Part model, mm, in its own coordinate system. Face numbers are marked on the shaded views. Give positions to 0.01 mm unless a question says otherwise; leave off trailing zeros. Order: outer loops, then holes, each group sorted by start corner. A loop starts at its lowest first (then second) coordinate and runs counter-clockwise, first axis right, second up. Notation, with made-up numbers: (88.25, 4) -> (102.25, 4) arc R23 cw to (102.25, 28) -> close; hole circle Ø9 at (79, 31.5). An arc over 180 degrees is marked (long way). Write item = value, one per line. Start each with the question number.
Item 1: Band-saw the part on D-D on z = 0. Write the cut outline in (x, y).
Item 2: Band-saw the part on A-A on x = -22. Write the cut outline in (y, z), plus the area to 4 significant figures.
Item 3: Pull direction Z, two halves, no side cores. Call the marked faces 1, 2, 3 and 4: +Z half, -Z half, draft (parallel to the pull), parting line (faces both ways), or undercut.
Item 4: Band-saw the part on C-C on y = -1.75. Write the cut outline in (x, z), plus the area to 3 significant figures.
Item 5: Band-saw the part on B-B on z = 37.5. Write the cut outline in (x, y).
Item 6: Drill centre lines: line 1 along X through (y, z) = (2.4, 0); line 2 along X through (y, z) = (0.75, 37.5); line 3 along Z through (x, y) = (-30, -4.5). Where is each one in solid material? Low to high.
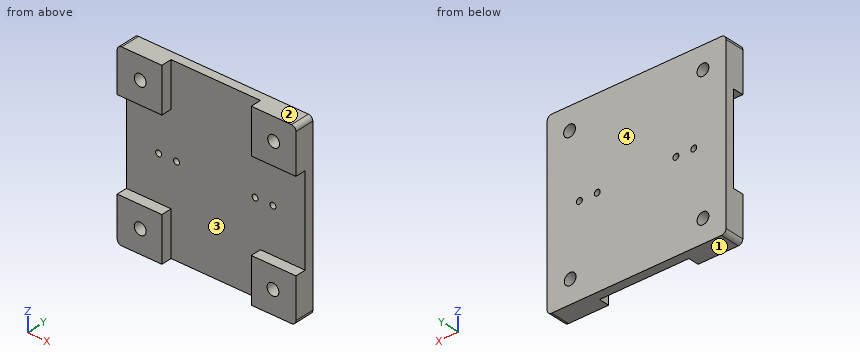
```python
from build123d import *

# Parameters (mm, degrees)
BOSS_EXTRUDE1_DEPTH  = 5
BOSS_EXTRUDE2_START  = 6
BOSS_EXTRUDE2_DEPTH  = 6
SKETCH1_3_R          = 1.65
CUT_EXTRUDE1_DEPTH   = 71.964779997
M6_CLEARANCE_HOLE2_D = 6.6


with BuildPart() as part:
    # Sketch1 → Boss-Extrude1 (new body)
    with BuildSketch(Plane(origin=(0, 0, 0), x_dir=(1, 0, 0), z_dir=(0, 1, 0))):
        with BuildLine():
            Line((-47.5, 50), (47.5, 50))
            ThreePointArc((47.5, 50), (49.267766953, 49.267766953), (50, 47.5))
            Line((50, 47.5), (50, -47.5))
            ThreePointArc((50, -47.5), (49.267766953, -49.267766953), (47.5, -50))
            Line((47.5, -50), (-47.5, -50))
            ThreePointArc((-47.5, -50), (-49.267766953, -49.267766953), (-50, -47.5))
            Line((-50, -47.5), (-50, 47.5))
            ThreePointArc((-50, 47.5), (-49.267766953, 49.267766953), (-47.5, 50))
        make_face()
    extrude(amount=BOSS_EXTRUDE1_DEPTH)

    # Sketch2 → Boss-Extrude2 (add)
    with BuildSketch(Plane.XZ.offset(BOSS_EXTRUDE2_START)):
        with BuildLine():
            Line((-25, 25), (-50, 25))
            Line((-50, 25), (-50, 47.5))
            ThreePointArc((-50, 47.5), (-49.267766953, 49.267766953), (-47.5, 50))
            Line((-47.5, 50), (-25, 50))
            Line((-25, 50), (-25, 25))
        make_face()
        with BuildLine():
            Line((25, 25), (50, 25))
            Line((50, 25), (50, 47.5))
            ThreePointArc((50, 47.5), (49.267766953, 49.267766953), (47.5, 50))
            Line((47.5, 50), (25, 50))
            Line((25, 50), (25, 25))
        make_face()
        with BuildLine():
            Line((25, -25), (50, -25))
            Line((50, -25), (50, -47.5))
            ThreePointArc((50, -47.5), (49.267766953, -49.267766953), (47.5, -50))
            Line((47.5, -50), (25, -50))
            Line((25, -50), (25, -25))
        make_face()
        with BuildLine():
            Line((-25, -25), (-50, -25))
            Line((-50, -25), (-50, -47.5))
            ThreePointArc((-50, -47.5), (-49.267766953, -49.267766953), (-47.5, -50))
            Line((-47.5, -50), (-25, -50))
            Line((-25, -50), (-25, -25))
        make_face()
    extrude(amount=-BOSS_EXTRUDE2_DEPTH)

    # Sketch1_3 → Cut-Extrude1 (cut, through all)
    with BuildSketch(Plane(origin=(0, 0, 0), x_dir=(1, 0, 0), z_dir=(0, 1, 0))):
        with Locations(Location((-32, 0, 0), (0, 0, 270))):
            Circle(SKETCH1_3_R)
        with Locations(Location((-22, 0, 0), (0, 0, 270))):
            Circle(SKETCH1_3_R)
        with Locations(Location((22, 0, 0), (0, 0, 270))):
            Circle(SKETCH1_3_R)
        with Locations(Location((32, 0, 0), (0, 0, 270))):
            Circle(SKETCH1_3_R)
    extrude(amount=CUT_EXTRUDE1_DEPTH, mode=Mode.SUBTRACT)

    # M6 Clearance Hole2 (through all)
    with Locations(Plane(origin=(0, 5, 0), x_dir=(1, 0, 0), z_dir=(0, 1, 0))):
        with Locations((-37.133883476, 37.133883476), (37.5, -37.5), (-37.133883476, -37.5), (37.133883476, 37.133883476)):
            Hole(M6_CLEARANCE_HOLE2_D / 2)


solid = part.part
```
Values found:
q1.outline = (-50, 0) -> (-33.65, 0) -> (-33.65, 5) -> (-50, 5) -> close; (-30.35, 0) -> (-23.65, 0) -> (-23.65, 5) -> (-30.35, 5) -> close; (-20.35, 0) -> (20.35, 0) -> (20.35, 5) -> (-20.35, 5) -> close; (23.65, 0) -> (30.35, 0) -> (30.35, 5) -> (23.65, 5) -> close; (33.65, 0) -> (50, 0) -> (50, 5) -> (33.65, 5) -> close
q2.outline = (0, -50) -> (5, -50) -> (5, -1.65) -> (0, -1.65) -> close; (0, 1.65) -> (5, 1.65) -> (5, 50) -> (0, 50) -> close
q2.area = 483.5 mm^2
q3.face_1 = -Z half
q3.face_2 = +Z half
q3.face_3 = undercut
q3.face_4 = draft
q4.outline = (-50, -47.5) arc R2.5 ccw to (-47.5, -50) -> (-25, -50) -> (-25, -25) -> (-50, -25) -> close; (-50, 25) -> (-25, 25) -> (-25, 50) -> (-47.5, 50) arc R2.5 ccw to (-50, 47.5) -> close; (25, -50) -> (47.5, -50) arc R2.5 ccw to (50, -47.5) -> (50, -25) -> (25, -25) -> close; (25, 25) -> (50, 25) -> (50, 47.5) arc R2.5 ccw to (47.5, 50) -> (25, 50) -> close; hole circle Ø6.6 at (-37.13, -37.13); hole circle Ø6.6 at (-37.13, 37.5); hole circle Ø6.6 at (37.13, -37.13); hole circle Ø6.6 at (37.5, 37.5)
q4.area = 2,360 mm^2
q5.outline = (-50, -6) -> (-40.43, -6) -> (-40.43, 5) -> (-50, 5) -> close; (-33.83, -6) -> (-25, -6) -> (-25, 0) -> (25, 0) -> (25, -6) -> (34.2, -6) -> (34.2, 5) -> (-33.83, 5) -> close; (40.8, -6) -> (50, -6) -> (50, 5) -> (40.8, 5) -> close
q6.line_1 = -50 to -33.65, -30.35 to -23.65, -20.35 to 20.35, 23.65 to 30.35, 33.65 to 50
q6.line_2 = -50 to -40.43, -33.83 to 34.2, 40.8 to 50
q6.line_3 = -50 to -25, 25 to 50
